from build123d import *

# Parameters (mm, degrees)
SFAZOWANIE1_SIZE = 1
SFAZOWANIE2_SIZE = 0.5


with BuildPart() as part:
    # Szkic1 → Obrót1 (revolve)
    with BuildSketch(Plane.XY, mode=Mode.PRIVATE) as obr_t1_sk:
        Polygon((0, 0), (0, 5), (0.6, 5), (0.6, 4.6), (1.7, 4.6), (1.7, 5), (11.2, 5), (11.2, 10.2), (31.2, 10.2), (31.2, 9.5), (65.2, 9.5), (65.2, 10.2), (85.2, 10.2), (85.2, 12.25), (88.2, 12.25), (88.2, 5), (97.7, 5), (97.7, 4.6), (98.8, 4.6), (98.8, 5), (99.4, 5), (99.4, 0), align=None)
    revolve(obr_t1_sk.sketch.rotate(Axis((-10.674656103, 0, 0), (1, 0, 0)), 90), axis=Axis((-10.674656103, 0, 0), (1, 0, 0)))

    # Sfazowanie1
    # the kernel refuses this chamfer: 1 mm, written as the material it takes off along each edge
    with BuildSketch(Plane(origin=(65.2, 0, 0), x_dir=(0, 0, 1), z_dir=(0, 1, 0))) as sfazowanie1_piece_1_section:
        Polygon((10.2 - SFAZOWANIE1_SIZE, 0), (10.2, SFAZOWANIE1_SIZE), (10.2, 0), align=None)
    sfazowanie1_piece_1 = revolve(axis=Axis((65.2, 0, 0), (1, 0, 0)), mode=Mode.PRIVATE)
    sfazowanie1_piece_1 = sfazowanie1_piece_1 - Plane(origin=(65.841981052, 0, 0), x_dir=(0, 0, 1), z_dir=(1, 0, 0)) * Cylinder(9.5, 41, mode=Mode.PRIVATE)
    add(sfazowanie1_piece_1, mode=Mode.SUBTRACT)
    with BuildSketch(Plane(origin=(31.2, 0, 0), x_dir=(0, 0, 1), z_dir=(0, 1, 0))) as sfazowanie1_piece_2_section:
        Polygon((10.2, -SFAZOWANIE1_SIZE), (10.2 - SFAZOWANIE1_SIZE, 0), (10.2, 0), align=None)
    sfazowanie1_piece_2 = revolve(axis=Axis((31.2, 0, 0), (1, 0, 0)), mode=Mode.PRIVATE)
    sfazowanie1_piece_2 = sfazowanie1_piece_2 - Plane(origin=(30.558018948, 0, 0), x_dir=(0, 0, 1), z_dir=(1, 0, 0)) * Cylinder(9.5, 41, mode=Mode.PRIVATE)
    add(sfazowanie1_piece_2, mode=Mode.SUBTRACT)
    with BuildSketch(Plane(origin=(88.2, 0, 0), x_dir=(0, 0, 1), z_dir=(0, 1, 0))) as sfazowanie1_piece_3:
        Polygon((12.25, -SFAZOWANIE1_SIZE), (12.25 - SFAZOWANIE1_SIZE, 0), (12.25, 0), align=None)
    revolve(axis=Axis((88.2, 0, 0), (1, 0, 0)), mode=Mode.SUBTRACT)
    with BuildSketch(Plane(origin=(11.2, 0, 0), x_dir=(0, 0, 1), z_dir=(0, 1, 0))) as sfazowanie1_piece_4:
        Polygon((10.2 - SFAZOWANIE1_SIZE, 0), (10.2, SFAZOWANIE1_SIZE), (10.2, 0), align=None)
    revolve(axis=Axis((11.2, 0, 0), (1, 0, 0)), mode=Mode.SUBTRACT)

    # Sfazowanie2
    sfazowanie2_edges = [part.edges().sort_by_distance(p)[0] for p in [
        (99.4, 0, -5),
        (0, 0, -5),
    ]]
    chamfer(sfazowanie2_edges, length=SFAZOWANIE2_SIZE)


solid = part.part
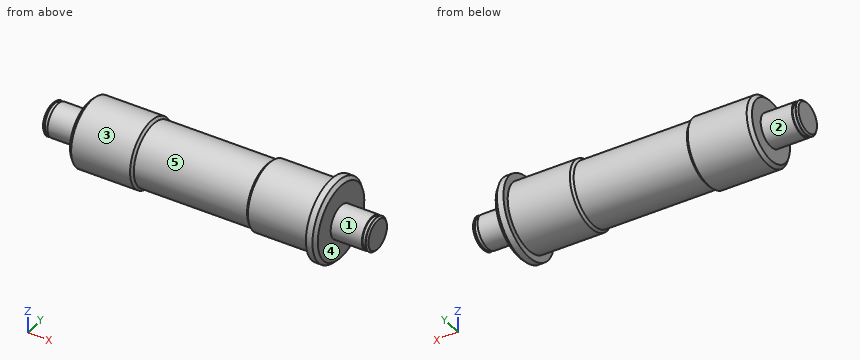
Geometry: final body of the model. Coordinates: model frame, mm. Face numbers are marked on the shaded views. A direction names the side the tool comes from. Give positions to 0.01 mm unless a question says otherwise; leave off trailing zeros. Order: outer loops, then holes, each group sorted by start corner. A loop starts at its lowest first (then second) coordinate and runs counter-clockwise, first axis right, second up. Notation, with made-up numbers: (60, 8.5) -> (75, 8.5) arc R28 cw to (75, 40.5) -> close; hole circle Ø4 at (-22.75, 7.25). An arc over 180 degrees is marked (long way). Answer as a JSON object with one key per item and string values.
Q1. Draft query along X for the marked faces 3, 4 and 5. Return one class per face: released by +X, released by -X, zero draft, split by the parting line, or undercut.
Entries:
{"face 3": "zero draft", "face 4": "released by +X", "face 5": "undercut"}
Q2. Material intervals for probe 1 along X at (y, z) = (6, -5.75); probe 2 along X at (y, z) = (-9.25, -3.25); probe 3 along X at (y, z) = (-10, 6.25), sorted ascending.
Entries:
{"probe 1": "x = 11.2 to 88.2", "probe 2": "x = 11.8 to 30.6, 65.8 to 88.2", "probe 3": "x = 85.2 to 87.66"}
Q3. Access query for the marked faces 1 and 2. Directions: +Z, -Z, +X, -X, +Y, -Y. A direction counts if a zero-diameter tool reaches every point of the face in a straight line with its end or side. Return the directions, or none.
Entries:
{"face 1": "+X", "face 2": "-X"}
Q4. Section B-B (x = 72.5). Output: boundary loops of the cut face in (y, z), plus the area to 3 significant figures.
Entries:
{"outline": "circle Ø20.4 at (0, 0)", "area": "327 mm^2"}
Q5. Section A-A (x = 40). Output: boundary loops of the cut face in (y, z).
Entries:
{"outline": "circle Ø19 at (0, 0)"}
Q6. First-contact query: pin 1 (6 mm diameter, centred on x = 15, y = 7, fed in from -Z); pin 2 (4 mm diameter, centred on x = 42, z = 1.5, fed in from +Y); pin 3 (5 mm diameter, centred on x = 56, y = -1, fed in from -Z). Flat tips, straight axial feed; report the tip coordinate or a pass-through.
Entries:
{"pin 1": "stops at z = -9.38", "pin 2": "stops at y = 9.5", "pin 3": "stops at z = -9.5"}
